```python
from build123d import *

# Parameters (mm, degrees)
F0_R     = 8.922134
F0_R_2   = 9.189262
F1_DEPTH = 13.208
F2_W     = 41.098034
F2_H     = 42.701147
F3_DEPTH = 17.78
F4_W     = 22.443607
F4_H     = 42.992625
F5_DEPTH = 32.766
F7_DEPTH = 42.672
F9_DEPTH = 18.288


with BuildPart() as f1:
    # F0 (on Front) → F1 (new body)
    with BuildSketch(Plane.XZ):
        Polygon((57.588355, 42.686574), (-63.061645, 42.686574), (-63.061645, 10.936574), (-39.022743, -18.62254), (33.549454, -18.62254), (57.588355, 10.936574), align=None)
        with Locations((-49.73989, 26.811574)):
            Circle(F0_R, mode=Mode.SUBTRACT)
        with Locations((39.919995, 26.811574)):
            Circle(F0_R_2, mode=Mode.SUBTRACT)
    extrude(amount=F1_DEPTH)

    # F2 (on Front) → F3 (join)
    with BuildSketch(Plane.XZ):
        with Locations((-1.89459, 21.350573)):
            Rectangle(F2_W, F2_H)
    extrude(amount=F3_DEPTH)

    # F4 (on Front) → F5 (join)
    with BuildSketch(Plane.XZ):
        with Locations((-11.221804, 21.496312)):
            Rectangle(F4_W, F4_H)
    extrude(amount=F5_DEPTH)

    # F6 (on Top) → F7 (join)
    with BuildSketch(Plane.XY):
        Polygon((0, -32.499507), (-22.443607, -32.499507), (-22.443607, -45.324426), (17.488524, -45.324426), (17.488524, -40.077869), (0, -40.077869), align=None)
    extrude(amount=F7_DEPTH)

    # F8 (on Top) → F9 (cut)
    with BuildSketch(Plane.XY):
        Polygon((0, -33.665407), (-22.443607, -33.665407), (-22.443607, -45.324426), (18.071475, -45.324426), (18.071475, -40.077869), (0, -40.077869), align=None)
    extrude(amount=F9_DEPTH, mode=Mode.SUBTRACT)


solid = f1.part
```
Input: part model. Units: mm. Frame: model coordinates. A direction names the side the tool comes from. Round coordinates to 2 decimals unless told otherwise and drop trailing zeros. Write each loop counter-clockwise with the first axis right and the second up, starting at its lowest first coordinate (ties: lowest second). Pieces come first, ordered by that corner, then holes. Notation, with made-up numbers: (-26.75, 9) -> (-16.75, 9) arc R24 ccw to (-16.75, 23) -> close; hole circle Ø8 at (84, -24.75). An arc over 180 degrees is marked (long way). Answer as CSV lines item,"result".
1. Section B-B (z = 38.5). Return the cut outline in (x, y).
Geometry says:
outline,"(-63.06, -13.21) -> (-22.44, -13.21) -> (-22.44, -45.32) -> (17.49, -45.32) -> (17.49, -40.08) -> (0, -40.08) -> (0, -17.78) -> (18.65, -17.78) -> (18.65, -13.21) -> (57.59, -13.21) -> (57.59, 0) -> (-63.06, 0) -> close"
2. Section A-A (x = 9). Return the cut outline in (y, z).
Geometry says:
outline,"(-45.32, 18.29) -> (-40.08, 18.29) -> (-40.08, 42.67) -> (-45.32, 42.67) -> close; (-17.78, 0) -> (-13.21, 0) -> (-13.21, -18.62) -> (0, -18.62) -> (0, 42.7) -> (-17.78, 42.7) -> close"
3. Contact query for flat-ended pins moving along their axis: P1, Ø16.5, axis at y = -23, z = 22, coming from the +X side; P2, Ø12, axis at y = -30, z = -3.5, coming from the +X side; P3, Ø3, axis at x = -36.5, z = 8.5, coming from the +Y side; P4, Ø14.5, axis at x = -43.5, y = -4.5, coming from the +Z side. Output: stop coordinate, or through.
Geometry says:
P1,"stops at x = 18.65"
P2,"stops at x = 0"
P3,"stops at y = 0"
P4,"stops at z = 42.69"
4. Section C-C (x = -4). Return the cut outline in (y, z), plus the area to 3 significant figures.
Geometry says:
outline,"(-45.32, 18.29) -> (-33.67, 18.29) -> (-33.67, 0) -> (-13.21, 0) -> (-13.21, -18.62) -> (0, -18.62) -> (0, 42.99) -> (-32.77, 42.99) -> (-32.77, 42.67) -> (-45.32, 42.67) -> close"
area,"1,980 mm^2"
5. Section D-D (z = 25). Return the cut outline in (x, y).
Geometry says:
outline,"(-63.06, -13.21) -> (-58.48, -13.21) -> (-58.48, 0) -> (-63.06, 0) -> close; (-41, -13.21) -> (-22.44, -13.21) -> (-22.44, -45.32) -> (17.49, -45.32) -> (17.49, -40.08) -> (0, -40.08) -> (0, -17.78) -> (18.65, -17.78) -> (18.65, -13.21) -> (30.91, -13.21) -> (30.91, 0) -> (-41, 0) -> close; (48.93, -13.21) -> (57.59, -13.21) -> (57.59, 0) -> (48.93, 0) -> close"
6. Reachability of faces 1 (the flat face through (17.489, -43, 30)), 2 (the flat face through (-7, -40, 42.672)), 3 (the flat face through (9, -17.78, 22)) from +Z, -Z, +X, -X, +Y, -Y: full face, straight path, thin tool, end or side. Return the list, or none.
Geometry says:
face 1,"+Z, -Z, +X, -Y"
face 2,"+Z, +X, -X, -Y"
face 3,"+Z, -Z, +X"
7. Ray query, L1, parallel to Y at x = -24, z = -3; L2, parallel to Z at x = 1.5, y = -12; L3, parallel to Y at x = -2, z = 11. Return the intervals inside material, ascending. Write a range as [from, to].
Geometry says:
L1,"y = [-13.21, 0]"
L2,"z = [-18.62, 42.7]"
L3,"y = [-33.67, 0]"
8. Mould query, pull axis Y, two halves, no side actions, for faces 4 (the flat face through (-3, -45.324, 30)), 5 (the flat face through (9, -40.078, 30)), 6 (the flat face through (38, -7, 42.687)). Classes: +Y half, -Y half, draft (parallel to the pull), parting line (faces both ways), or undercut.
Geometry says:
face 4,"-Y half"
face 5,"undercut"
face 6,"draft"
